Could you check a few things on this model? Use its own coordinates, in mm. Coordinates: 2 decimals unless noted, no trailing zeros. Loops run counter-clockwise (first coordinate to the right, second up) from the corner with the lowest first, then second, coordinate; pieces in that order, holes last.
1) Imagine slicing it at D-D on x = -4. Please give me the cut outline in (y, z).
2) Thinking about a two-plate mould opening in X: for faces 1 (the face through (-2.2, 0, -2.2)), 2 (the face through (1.08, 3.94, 4.88)), 3 (the face through (0.596, 4.19, 2.685)), which applies, released by +X, released by -X, zero draft, split by the parting line, or undercut?
3) Imagine slicing it at C-C on y = 2.75. Please give me the cut outline in (x, z), plus the area to 3 significant figures.
4) Will these pins go through, and if not, where does the flat tip stop? P1, Ø2, axis at y = 7, z = 4, coming from the +X side; P2, Ø3, axis at y = 1.5, z = 3.5, coming from the +X side; P3, Ø2, axis at y = 6, z = 4, coming from the -X side.
5) If I drill on line 1 along Z through (x, y) = (0, 2.5); line 2 along Z through (x, y) = (1.75, 7.25); line 3 along Y through (x, z) = (-4.25, 2.25), over which ranges is the centre line in solid material (lowest first)?
Autodesk Inventor part; units mm, degrees
ref_plane "YZ Plane" through (0, 0, 0) normal (1, 0, 0) x (0, 1, 0)
ref_plane "XZ Plane" through (0, 0, 0) normal (0, 1, 0) x (-1, 0, 0)
ref_plane "XY Plane" through (0, 0, 0) normal (0, 0, 1) x (1, 0, 0)
sketch "Sketch1" plane through (0, 0, 0) normal (0, 1, 0) x (-1, 0, 0)
  circle A0 centre (0, 0) radius 2.75
  circle A1 centre (0, 0) radius 5
  dimension "d0" = 5.5
  dimension "d1" = 10
extrude "Extrusion1" add sketch "Sketch1" along normal blind 8.5
sketch "Sketch2" plane through (0, 8.5, 0) normal (0, 1, 0) x (1, 0, 0)
  circle A0 centre (0, 0) radius 2.75
  circle A1 centre (0, 0) radius 5
  circle A2 centre (0, 0) radius 3.75
  dimension "d4" = 1
extrude "Extrusion2" cut sketch "Sketch2" against normal blind 0.5 contours A1
chamfer "Chamfer1" distance 0.5 angle 45 1 edges at (-3.75, 8.5, 0)
properties part number "m5_9mm"
Filled in:
1. outline: (0, -3) - (8, -3) - (8, 3) - (0, 3) - close
2. face 1: zero draft
2. face 2: split by the parting line
2. face 3: undercut
3. outline: circle Ø10 at (0, 0); hole circle Ø5.5 at (0, 0)
3. area: 54.8 mm2
4. P1: stops at x = 4
4. P2: stops at x = 4.58
4. P3: stops at x = -4
5. line 1: z = -5 to -2.75, 2.75 to 5
5. line 2: z = -4.68 to -2.12, 2.12 to 4.68
5. line 3: y = 0 to 8
